```python
from build123d import *

# Parameters (mm, degrees)
F1_DEPTH = 25


with BuildPart() as f1:
    # F0 (on Front) → F1 (new body)
    with BuildSketch(Plane.XZ):
        with BuildLine():
            Line((-124.571604, -610.826684), (395.039996, -610.826684))
            Line((395.039996, -610.826684), (0.605091, -394.213883))
            Line((0.605091, -394.213883), (0.605091, -344.213883))
            Line((0.605091, -344.213883), (31.970073, -281.634031))
            Line((31.970073, -281.634031), (-39.549758, -245.788336))
            Line((-39.549758, -245.788336), (1.378216, -164.12827))
            ThreePointArc((1.378216, -164.12827), (2.961033, -159.771238), (3.498259, -155.166846))
            Line((3.498259, -155.166846), (3.498259, 192.592175))
            ThreePointArc((3.498259, 192.592175), (0.517232, 203.097153), (-7.537197, 210.470568))
            Line((-7.537197, 210.470568), (-89.129627, 251.382462))
            Line((-89.129627, 251.382462), (-53.27145, 322.896036))
            Line((-53.27145, 322.896036), (-124.571604, 358.6472))
            Line((-124.571604, 358.6472), (-124.571604, -610.826684))
        make_face()
    extrude(amount=F1_DEPTH)


solid = f1.part
```
Input: part model. Units: mm. Frame: model coordinates. A direction names the side the tool comes from. Coordinates: 2 decimals unless noted, no trailing zeros. Write each loop counter-clockwise with the first axis right and the second up, starting at its lowest first coordinate (ties: lowest second). Pieces come first, ordered by that corner, then holes. Notation, with made-up numbers: (-11, 57.25) -> (2, 57.25) arc R25 ccw to (2, 85.25) -> close; hole circle Ø10 at (17, 41.25). An arc over 180 degrees is marked (long way). Answer as a JSON object with one key per item and string values.
1. Material intervals for line 1 (X direction, y = -12.75, z = 190); line 2 (Z direction, x = -22.5, y = -2.5); line 3 (Z direction, x = 0, y = -15.5), sorted ascending. Write a range as from..to.
Result set:
{"line 1": "x = -124.57..3.5", "line 2": "z = -610.83..-254.33, -211.77..217.97", "line 3": "z = -610.83..-265.61, -166.88..203.89"}
2. Mould query, pull axis Z, two halves, no side actions, for faces 1 (the face through (-124.572, -12, -119)), 2 (the face through (132, -12, -610.827)), 3 (the face through (-71.45, -12.32, 286.64)). Classes: released by +Z, released by -Z, zero draft, split by the parting line, or undercut.
Result set:
{"face 1": "zero draft", "face 2": "released by -Z", "face 3": "undercut"}
3. Section A-A on x = -69.5. Return the cut outline in (y, z).
Result set:
{"outline": "(-25, -610.83) -> (0, -610.83) -> (0, 241.54) -> (-25, 241.54) -> close; (-25, 290.53) -> (0, 290.53) -> (0, 331.03) -> (-25, 331.03) -> close"}
4. First-contact query: P1, Ø1.5, axis at x = -28.5, y = -21, coming from the +Z side; P2, Ø7.5, axis at y = -13, z = 76.5, coming from the +X side. Flat tips, straight axial feed; report the tip coordinate or a pass-through.
Result set:
{"P1": "stops at z = 221.36", "P2": "stops at x = 3.5"}
5. Section C-C on z = 157.5. Return the cut outline in (x, y).
Result set:
{"outline": "(-124.57, -25) -> (3.5, -25) -> (3.5, 0) -> (-124.57, 0) -> close"}
6. Access query for faces 4 (the face through (3.498, -12, 16)), 5 (the face through (-20, 0, -267)), 6 (the face through (-19.372, -12.325, -205.53)). Directions: +Z, -Z, +X, -X, +Y, -Y. A direction counts if a zero-diameter tool reaches every point of the face in a straight line with its end or side. Return the directions, or none.
Result set:
{"face 4": "+Z, +X, +Y, -Y", "face 5": "+Z, -Z, +X, -X, +Y", "face 6": "+X, +Y, -Y"}
7. Section B-B on y = -8.25. Return the cut outline in (x, z), then the cut area to 3 significant figures.
Result set:
{"outline": "(-124.57, -610.83) -> (395.04, -610.83) -> (0.61, -394.21) -> (0.61, -344.21) -> (31.97, -281.63) -> (-39.55, -245.79) -> (1.38, -164.13) arc R20 ccw to (3.5, -155.17) -> (3.5, 192.59) arc R20 ccw to (-7.54, 210.47) -> (-89.13, 251.38) -> (-53.27, 322.9) -> (-124.57, 358.65) -> close", "area": "154,000 mm2"}
8. Section D-D on x = 114. Return the cut outline in (y, z).
Result set:
{"outline": "(-25, -610.83) -> (0, -610.83) -> (0, -456.49) -> (-25, -456.49) -> close"}
